Here's how the part is built. I have some questions about the finished solid (model axes, mm). A direction names the side the tool comes from. Coordinates: 2 decimals unless noted, no trailing zeros. Write each loop counter-clockwise with the first axis right and the second up, starting at its lowest first coordinate (ties: lowest second). Pieces come first, ordered by that corner, then holes.
Item 1: I want a section at C-C (x = 2.4). Count the separate pieces of the cut face and the enclosed holes in it, and give its area (3 significant figures).
Item 2: I want a section at B-B (z = -62.5). Please give me the cut outline in (x, y), and give its area (4 significant figures).
Item 3: I'm going to push flat-ended pins straight in: P1, Ø1.5, axis at x = 2, y = 3, coming from the -Z side; P2, Ø12, axis at y = 22, z = 4.5, coming from the -X side. Where does each tip first touch, or does it pass through?
Item 4: For faces 5 (the face through (3, -22.5, 9)), 6 (the face through (3, 25, 88)), 7 (the face through (3, -33, 10)), which set-ups out of +Z, -Z, +X, -X, +Y, -Y let a thin tool reach every point of the face, with its end or its side?
Item 5: I want a section at A-A (z = 43). Please give me the cut outline in (x, y), and give its area (4 significant figures).
Item 6: Please list where these lines run through material, in increasing order: line 1 (Z direction, x = 4, y = -31.5); line 2 (Y direction, x = 2.95, z = -58.5); line 3 (Y direction, x = 4.2, z = -2.5).
Item 7: If we mould it in two halves opening along Y, with no side actions, what happens to faces 1 (the face through (3, 32, 50)), 2 (the face through (3, 0, -87)), 3 (the face through (3, 5, -85)), 4 (the face through (3, -30, -40))? For each: pulls with the +Y half, pulls with the -Y half, needs draft (parallel to the pull), parting line crosses it, or undercut.
from build123d import *

# Parameters (mm, degrees)
ESQUISSE1_W             = 180
ESQUISSE1_H             = 70
BOSS_EXTRU_1_DEPTH      = 5
ESQUISSE2_W             = 165
ESQUISSE2_H             = 2.5
ENL_V_MAT_EXTRU_1_DEPTH = 5
ESQUISSE3_W             = 5
ESQUISSE3_H             = 10
ESQUISSE3_W_2           = 20
ESQUISSE3_H_2           = 5
ENL_V_MAT_EXTRU_2_DEPTH = 5
ESQUISSE4_W             = 2
ESQUISSE4_H             = 30
ENL_V_MAT_EXTRU_3_DEPTH = 5


with BuildPart() as part:
    # Esquisse1 → Boss.-Extru.1 (new body)
    with BuildSketch(Plane(origin=(0, 0, 0), x_dir=(0, 0, -1), z_dir=(1, 0, 0))):
        Rectangle(ESQUISSE1_W, ESQUISSE1_H)
    extrude(amount=BOSS_EXTRU_1_DEPTH)

    # Esquisse2 → Enlèv. mat.-Extru.1 (cut)
    with BuildSketch(Plane(origin=(5, 0, 0), x_dir=(0, 0, -1), z_dir=(1, 0, 0))):
        with Locations((-7.5, -23.75)):
            Rectangle(ESQUISSE2_W, ESQUISSE2_H)
    extrude(amount=-ENL_V_MAT_EXTRU_1_DEPTH, mode=Mode.SUBTRACT)

    # Esquisse3 → Enlèv. mat.-Extru.2 (cut)
    with BuildSketch(Plane(origin=(5, 0, 0), x_dir=(0, 0, -1), z_dir=(1, 0, 0))):
        with Locations((-87.5, 30)):
            Rectangle(ESQUISSE3_W, ESQUISSE3_H)
        with Locations((-87.5, 5)):
            Rectangle(ESQUISSE3_W, ESQUISSE3_H)
        with Locations((87.5, 30)):
            Rectangle(ESQUISSE3_W, ESQUISSE3_H)
        with Locations((87.5, 5)):
            Rectangle(ESQUISSE3_W, ESQUISSE3_H)
        with Locations((-40, 32.5)):
            Rectangle(ESQUISSE3_W_2, ESQUISSE3_H_2)
        with Locations((40, 32.5)):
            Rectangle(ESQUISSE3_W_2, ESQUISSE3_H_2)
        with Locations((0, 32.5)):
            Rectangle(ESQUISSE3_W_2, ESQUISSE3_H_2)
        with Locations((-40, -32.5)):
            Rectangle(ESQUISSE3_W_2, ESQUISSE3_H_2)
        with Locations((0, -32.5)):
            Rectangle(ESQUISSE3_W_2, ESQUISSE3_H_2)
        with Locations((40, -32.5)):
            Rectangle(ESQUISSE3_W_2, ESQUISSE3_H_2)
    extrude(amount=-ENL_V_MAT_EXTRU_2_DEPTH, mode=Mode.SUBTRACT)

    # Esquisse4 → Enlèv. mat.-Extru.3 (cut)
    with BuildSketch(Plane(origin=(5, 0, 0), x_dir=(0, 0, -1), z_dir=(1, 0, 0))):
        with Locations((32, 5)):
            Rectangle(ESQUISSE4_W, ESQUISSE4_H)
        with Locations((39, 5)):
            Rectangle(ESQUISSE4_W, ESQUISSE4_H)
        with Locations((25, 5)):
            Rectangle(ESQUISSE4_W, ESQUISSE4_H)
        with Locations((18, 5)):
            Rectangle(ESQUISSE4_W, ESQUISSE4_H)
        with Locations((11, 5)):
            Rectangle(ESQUISSE4_W, ESQUISSE4_H)
        with Locations((4, 5)):
            Rectangle(ESQUISSE4_W, ESQUISSE4_H)
        with Locations((-3, 5)):
            Rectangle(ESQUISSE4_W, ESQUISSE4_H)
        with Locations((-10, 5)):
            Rectangle(ESQUISSE4_W, ESQUISSE4_H)
        with Locations((-17, 5)):
            Rectangle(ESQUISSE4_W, ESQUISSE4_H)
        with Locations((-24, 5)):
            Rectangle(ESQUISSE4_W, ESQUISSE4_H)
    extrude(amount=-ENL_V_MAT_EXTRU_3_DEPTH, mode=Mode.SUBTRACT)


solid = part.part
Answer:
1. separate pieces: 1
1. enclosed holes: 10
1. area: 10,800 mm2
2. outline: (0, -35) - (5, -35) - (5, -25) - (0, -25) - close; (0, -22.5) - (5, -22.5) - (5, 35) - (0, 35) - close
2. area: 337.5 mm2
3. P1: stops at z = -85
3. P2: stops at x = 0
4. face 5: +Z, +X, -X
4. face 6: +Z, +X, -X, +Y
4. face 7: +X, -X, -Y
5. outline: (0, -30) - (5, -30) - (5, -25) - (0, -25) - close; (0, -22.5) - (5, -22.5) - (5, 30) - (0, 30) - close
5. area: 287.5 mm2
6. line 1: z = -90 to -50, -30 to -10, 10 to 30, 50 to 90
6. line 2: y = -35 to -25, -22.5 to 35
6. line 3: y = -30 to -25, -22.5 to 30
7. face 1: needs draft
7. face 2: undercut
7. face 3: undercut
7. face 4: pulls with the -Y half
